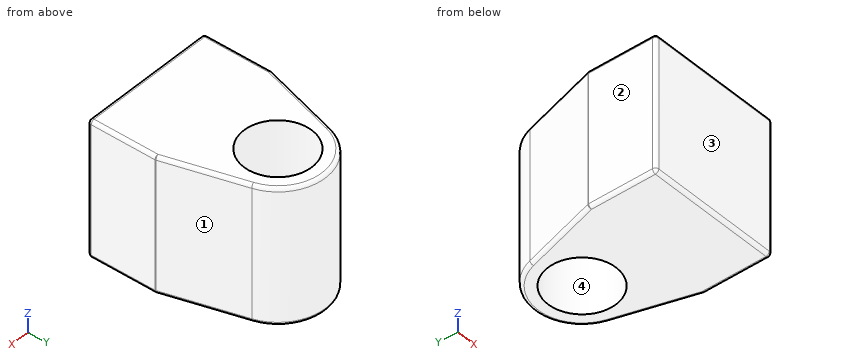
```python
from build123d import *

# Parameters (mm, degrees)
SKETCH_1_R      = 5
EXTRUDE_1_DEPTH = 20
FILLET_1_R      = 0.5


with BuildPart() as part:
    # 草图1 → 凸台-拉伸1 (new body)
    with BuildSketch(Plane.XY):
        with BuildLine():
            Line((6.729794889, 16.426099883), (10, 5))
            Line((10, 5), (10, -5))
            Line((10, -5), (-10, -5))
            Line((-10, -5), (-10, 5))
            Line((-10, 5), (-6.729794889, 16.426099883))
            ThreePointArc((-6.729794889, 16.426099883), (0, 21.5), (6.729794889, 16.426099883))
        make_face()
        with Locations((0, 14.5)):
            Circle(SKETCH_1_R, mode=Mode.SUBTRACT)
    extrude(amount=EXTRUDE_1_DEPTH)

    # 圆角1
    fillet_1_edges = [part.edges().sort_by_distance(p)[0] for p in [
        (10, -5, 10),
        (-10, -5, 10),
        (-10, 5, 10),
        (10, 5, 10),
        (0, 21.5, 20),
        (-8.364897444, 10.713049941, 20),
        (-10, 0, 20),
        (0, -5, 20),
        (10, 0, 20),
        (0, -5, 0),
        (-10, 0, 0),
        (-8.364897444, 10.713049941, 0),
        (0, 21.5, 0),
        (8.364897444, 10.713049941, 0),
        (10, 0, 0),
        (8.364897444, 10.713049941, 20),
    ]]
    fillet(fillet_1_edges, radius=FILLET_1_R)


solid = part.part
```
Work out the finished part from the listing and answer in its coordinate system (mm). Face numbers are marked on the shaded views. Coordinates: 2 decimals unless noted, no trailing zeros. Loops run counter-clockwise (first coordinate to the right, second up) from the corner with the lowest first, then second, coordinate; pieces in that order, holes last. Notation, with made-up numbers: M -5.75,-38 L 17.25,-38 A27 ccw 17.25,-21 Z; hole C 71.25,3.5 d9. An arc over 180 degrees is marked long. Use CSV: the item, a comma, the result in double quotes. Start each with the question number.
(1) Consider line 1 (Y direction, x = 0, z = 10.75); line 2 (Y direction, x = -2.25, z = 15); line 3 (X direction, y = 17.5, z = 2.5). Determine where each line is inside the solid, lowest interval first.
(2) Given pin 1 Ø1.5 at (y, z) = (12.5, 13) entering from -X; pin 2 Ø1 at (x, y) = (-4, 13.5) entering from +Z, each flat-ended and moving along its own axis, determine where each tip first touches the part or whether it passes through.
(3) For a pull along Y with two mould halves and no side action, classify the marked faces 1, 2, 3 and 4 as +Y half, -Y half, draft (parallel to the pull), parting line (faces both ways), or undercut.
(4) Find section B-B, the plane x = 0. Give the vertices of the cut face in (y, z), then the cut area to 3 significant figures.
(5) Find section A-A, the plane z = 18.25. Give the vertices of the cut face in (x, y), then the cut area to 3 significant figures.
Recorded:
1,line 1,"y = -5 to 9.5, 19.5 to 21.5"
1,line 2,"y = -5 to 10.03, 18.97 to 21.13"
1,line 3,"x = -6.32 to -4, 4 to 6.32"
2,pin 1,"stops at x = -8.07"
2,pin 2,"passes through"
3,face 1,"+Y half"
3,face 2,"draft"
3,face 3,"-Y half"
3,face 4,"undercut"
4,outline,"M -5,0.5 A0.5 ccw -4.5,0 L 9.5,0 L 9.5,20 L -4.5,20 A0.5 ccw -5,19.5 Z; M 19.5,0 L 21,0 A0.5 ccw 21.5,0.5 L 21.5,19.5 A0.5 ccw 21,20 L 19.5,20 Z"
4,area,"330 mm^2"
5,outline,"M -10,-4.5 A0.5 ccw -9.5,-5 L 9.5,-5 A0.5 ccw 10,-4.5 L 10,4.93 A0.5 ccw 9.98,5.07 L 6.73,16.43 A7 ccw -6.73,16.43 L -9.98,5.07 A0.5 ccw -10,4.93 Z; hole C 0,14.5 d10"
5,area,"363 mm^2"
